```python
from build123d import *

# Parameters (mm, degrees)
F1_DEPTH   = 28
F2_R       = 1.65
F3_DEPTH   = 1.75
F1_FACE1_W = 28
F1_FACE1_H = 1.75
F4_REACH   = 50.8712690127


with BuildPart() as f1:
    # F0 (on Right) → F1 (new body)
    with BuildSketch(Plane.YZ):
        with BuildLine():
            Line((-3, 35), (0, 35))
            Line((0, 35), (-10.1456508905, 9.0044083693))
            Line((-10.1456508905, 9.0044083693), (-10.1456508905, 0))
            Line((-10.1456508905, 0), (7.9644151033, 0))
            Line((7.9644151033, 0), (19.6633343933, 28.2374824987))
            ThreePointArc((19.6633343933, 28.2374824987), (19.8121032451, 29.121794497), (19.559512125, 29.9822232317))
            ThreePointArc((19.559512125, 29.9822232317), (18.9135949962, 30.766804474), (18.0350819326, 31.2776777068))
            Line((18.0350819326, 31.2776777068), (3, 36.75))
            Line((3, 36.75), (0, 36.75))
            Line((0, 36.75), (-3, 36.75))
            Line((-3, 36.75), (-3, 35))
        make_face()
        with BuildLine():
            Line((-8.6863745263, 9.0319523177), (1.4485264153, 35))
            Line((1.4485264153, 35), (3, 35))
            Line((3, 35), (8.0000780063, 33.1801204367))
            Line((8.0000780063, 33.1801204367), (9.1758168143, 32.7521865073))
            Line((9.1758168143, 32.7521865073), (16.3991077878, 30.1231235995))
            ThreePointArc((16.3991077878, 30.1231235995), (17.5457217574, 29.0491606036), (17.5627670801, 27.4782278969))
            Line((17.5627670801, 27.4782278969), (6.9034435496, 1.75))
            Line((6.9034435496, 1.75), (-3.6685321031, 1.75))
            Line((-3.6685321031, 1.75), (-5.0215659125, 1.75))
            Line((-5.0215659125, 1.75), (-8.6863745263, 1.75))
            Line((-8.6863745263, 1.75), (-8.6863745263, 9.0319523177))
        make_face(mode=Mode.SUBTRACT)
        Polygon((9.1758168143, 32.7521865073), (8.0000780063, 33.1801204367), (-5.0215659125, 1.75), (-3.6685321031, 1.75), align=None)
    extrude(amount=F1_DEPTH)

    # F2 (on face) → F3 (join)
    with BuildSketch(Plane.XY.offset(36.75)):
        with BuildLine():
            Line((0, -3), (0, 3))
            ThreePointArc((0, 3), (-3.6457513111, 2.215250437), (-6.6457513111, 0))
            ThreePointArc((-6.6457513111, 0), (-7.6807421272, -4.5659302006), (-3.673363624, -6.9866412778))
            ThreePointArc((-3.673363624, -6.9866412778), (-1.0583554341, -5.7104846888), (0, -3))
        make_face()
        with Locations((-4, -3)):
            Circle(F2_R, mode=Mode.SUBTRACT)
        with BuildLine():
            ThreePointArc((34.6457513111, 0), (31.6457513111, 2.215250437), (28, 3))
            Line((28, 3), (28, -3))
            ThreePointArc((28, -3), (29.0583554341, -5.7104846888), (31.673363624, -6.9866412778))
            ThreePointArc((31.673363624, -6.9866412778), (35.6807421272, -4.5659302006), (34.6457513111, 0))
        make_face()
        with Locations((32, -3)):
            Circle(F2_R, mode=Mode.SUBTRACT)
    extrude(amount=-F3_DEPTH)

    f4_end = Plane(origin=(14, -5.0728254453, 22.0022041847), x_dir=(0, -0.3635745105, -0.9315651213), z_dir=(0, -0.9315651213, 0.3635745105))
    # F1_face1 (on face) → F4 (cut, up to a plane its end follows)
    with BuildSketch(Plane(origin=(14, -3, 35.875), x_dir=(1, 0, 0), z_dir=(0, -1, 0))):
        Rectangle(F1_FACE1_W, F1_FACE1_H)
    f4_long = extrude(amount=-F4_REACH, mode=Mode.PRIVATE)
    add(split(f4_long, bisect_by=f4_end, keep=Keep.TOP, mode=Mode.PRIVATE), mode=Mode.SUBTRACT)


solid = f1.part
```
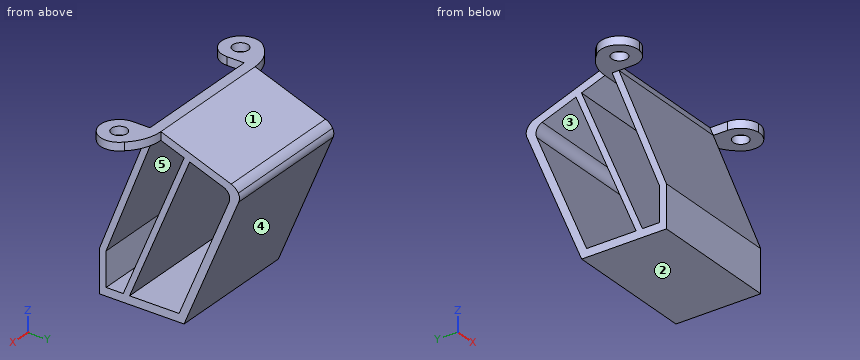
For this review, take the finished solid that the model builds, in its own axes (mm). Face numbers are marked on the shaded views. A direction names the side the tool comes from. Coordinates: 2 decimals unless noted, no trailing zeros. Loops run counter-clockwise (first coordinate to the right, second up) from the corner with the lowest first, then second, coordinate; pieces in that order, holes last.
1. For line 1 (Y direction, x = 15.5, z = 22); line 2 (Y direction, x = 13, z = 13.5); line 3 (Z direction, x = 17, y = 11.5), list the stretches that pass through material, from the lowest coordinate up.
2. Add section D-D, the plane x = -1. Give the boundary of the cut face in (y, z).
3. Add section C-C, the plane y = 6. Give the boundary of the cut face in (x, z), then the cut area to 3 significant figures.
4. Insertion check: P1, Ø0.9, axis at y = -1.5, z = 36, coming from the +X side; P2, Ø0.9, axis at y = -1, z = 35.5, coming from the -X side; P3, Ø9, axis at y = 0.5, z = 22.5, coming from the -X side; P4, Ø2, axis at x = 32, y = -3, coming from the +Z side. Each pin has a flat end and moves straight along its axis. Give the tip position at first contact, or say it passes through.
5. Add section A-A, the plane x = 26. Give the boundary of the cut face in (y, z), then the cut area to 3 significant figures.
6. For the marked faces 4 and 5, list the 3-axis set-ups (+Z, -Z, +X, -X, +Y, -Y) from which the entire face can be reached by the end or side of a thin tool; tool diameter is ignored.
7. Add section B-B, the plane z = 11. Give the boundary of the cut face in (x, y).
8. Mouldability with a two-part tool opening along Y and no side actions: class the marked faces 1, 2 and 3 as +Y half, -Y half, draft (parallel to the pull), parting line (faces both ways), or undercut.
Result:
1. line 1: y = -5.07 to -3.63, 3.37 to 4.72, 15.29 to 17.08
1. line 2: y = -8.39 to -6.94, -0.15 to 1.2, 11.77 to 13.56
1. line 3: z = 8.53 to 12.84, 31.91 to 33.66
2. outline: (-5.65, 35) - (2.94, 35) - (2.94, 36.75) - (-5.65, 36.75) - close
3. outline: (0, 0) - (28, 0) - (28, 1.75) - (0, 1.75) - close; (0, 25.09) - (28, 25.09) - (28, 28.35) - (0, 28.35) - close; (0, 33.91) - (28, 33.91) - (28, 35.66) - (0, 35.66) - close
3. area: 189 mm2
4. P1: stops at x = 35.86
4. P2: stops at x = -7.69
4. P3: stops at x = 0
4. P4: passes through
5. outline: (-10.15, 0) - (7.96, 0) - (19.66, 28.24) arc R2 ccw to (19.56, 29.98) arc R2.88 ccw to (18.04, 31.28) - (3, 36.75) - (0.68, 36.75) - (-10.15, 9) - close; hole (-8.69, 1.75) - (-5.02, 1.75) - (8, 33.18) - (3, 35) - (1.45, 35) - (-8.69, 9.03) - close; hole (-3.67, 1.75) - (6.9, 1.75) - (17.56, 27.48) arc R2 ccw to (16.4, 30.12) - (9.18, 32.75) - close
5. area: 206 mm2
6. face 4: -Z, +X, -X, +Y
6. face 5: +X, -X
7. outline: (0, -9.37) - (28, -9.37) - (28, -7.92) - (0, -7.92) - close; (0, -1.19) - (28, -1.19) - (28, 0.16) - (0, 0.16) - close; (0, 10.74) - (28, 10.74) - (28, 12.52) - (0, 12.52) - close
8. face 1: +Y half
8. face 2: draft
8. face 3: undercut
